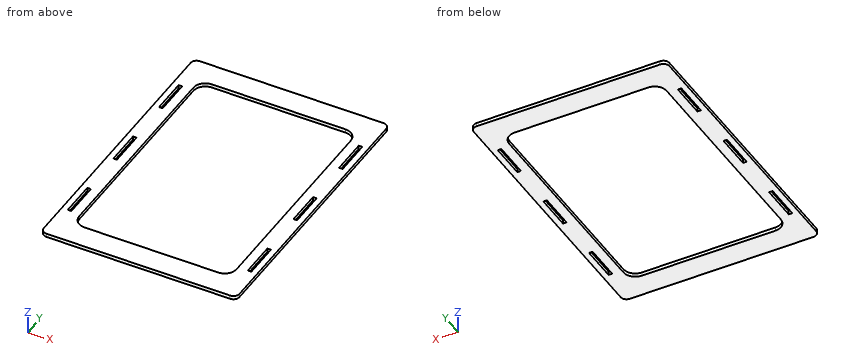
```python
from build123d import *

# Parameters (mm, degrees)
F0_W     = 164
F0_H     = 235
F0_W_2   = 3
F0_H_2   = 30
F0_W_3   = 132
F0_H_3   = 195
F1_DEPTH = 3
F2_R     = 5
F3_R     = 10


with BuildPart() as f1:
    # F0 (on Top) → F1 (new body)
    with BuildSketch(Plane.XY):
        with Locations((77, 112.5)):
            Rectangle(F0_W, F0_H)
        with Locations((1.5, 42.5)):
            Rectangle(F0_W_2, F0_H_2, mode=Mode.SUBTRACT)
        with Locations((152.5, 42.5)):
            Rectangle(F0_W_2, F0_H_2, mode=Mode.SUBTRACT)
        with Locations((1.5, 112.5)):
            Rectangle(F0_W_2, F0_H_2, mode=Mode.SUBTRACT)
        with Locations((1.5, 182.5)):
            Rectangle(F0_W_2, F0_H_2, mode=Mode.SUBTRACT)
        with Locations((77, 112.5)):
            Rectangle(F0_W_3, F0_H_3, mode=Mode.SUBTRACT)
        with Locations((152.5, 112.5)):
            Rectangle(F0_W_2, F0_H_2, mode=Mode.SUBTRACT)
        with Locations((152.5, 182.5)):
            Rectangle(F0_W_2, F0_H_2, mode=Mode.SUBTRACT)
    extrude(amount=F1_DEPTH)

    # F2
    f2_edges = [f1.edges().sort_by_distance(p)[0] for p in [
        (-5, 230, 1.5),
        (159, 230, 1.5),
        (159, -5, 1.5),
        (-5, -5, 1.5),
    ]]
    fillet(f2_edges, radius=F2_R)

    # F3
    f3_edges = [f1.edges().sort_by_distance(p)[0] for p in [
        (11, 210, 1.5),
        (143, 210, 1.5),
        (143, 15, 1.5),
        (11, 15, 1.5),
    ]]
    fillet(f3_edges, radius=F3_R)


solid = f1.part
```
CAD build for the part. Positions are in the model's coordinates, mm. Give positions to 0.01 mm unless a question says otherwise; leave off trailing zeros. Write each loop counter-clockwise with the first axis right and the second up, starting at its lowest first coordinate (ties: lowest second). Pieces come first, ordered by that corner, then holes. Notation, with made-up numbers: M -39,28.25 L 1,28.25 A10 ccw 1,34.25 Z; hole C 83.5,-28.75 d6. An arc over 180 degrees is marked long. Return JSON: item names as keys, results as strings. Group by question number.
(1) Band-saw the part on B-B (x = 121). Give the cut face in (y, z), and give its area (3 significant figures).
(2) Band-saw the part on A-A (y = 72). Give the cut face in (x, z), and give its area (3 significant figures).
(3) Drill centre lines: L1, parallel to X at y = 50.5, z = 2.4; L2, parallel to X at y = 163.5, z = 2.6; L3, parallel to Y at x = 83, z = 0.3. Where is each one in solid material? Low to high. Write a range as [from, to].
(4) Band-saw the part on D-D (z = 1.85). State how many separate pieces and enclosed holes the cut face has, and give its area (3 significant figures).
(5) Band-saw the part on C-C (y = 175.5). Give the cut face in (x, z), and give its area (3 significant figures).
Entries:
{
 "1": {"outline": "M -5,0 L 15,0 L 15,3 L -5,3 Z; M 210,0 L 230,0 L 230,3 L 210,3 Z", "area": "120 mm^2"},
 "2": {"outline": "M -5,0 L 11,0 L 11,3 L -5,3 Z; M 143,0 L 159,0 L 159,3 L 143,3 Z", "area": "96.0 mm^2"},
 "3": {"L1": "x = [-5, 0], [3, 11], [143, 151], [154, 159]", "L2": "x = [-5, 11], [143, 159]", "L3": "y = [-5, 15], [210, 230]"},
 "4": {"separate pieces": "1", "enclosed holes": "7", "area": "12,300 mm^2"},
 "5": {"outline": "M -5,0 L 0,0 L 0,3 L -5,3 Z; M 3,0 L 11,0 L 11,3 L 3,3 Z; M 143,0 L 151,0 L 151,3 L 143,3 Z; M 154,0 L 159,0 L 159,3 L 154,3 Z", "area": "78.0 mm^2"}
}
